Can you work these out from the model? Positions are in its coordinate system, mm. Coordinates: 2 decimals unless noted, no trailing zeros. Loops run counter-clockwise (first coordinate to the right, second up) from the corner with the lowest first, then second, coordinate; pieces in that order, holes last.
```python
from build123d import *

# Parameters (mm, degrees)
FILLET2_R = 10


# Read off the part's stored shape, not the designer's step: Revolve-Thin1
with BuildPart() as part:
    # Revolve-Thin1 outline → Revolve-Thin1 (revolve)
    with BuildSketch(Plane.YX):
        with BuildLine():
            ThreePointArc((20.809194043, 175.40901311), (18.540551824, 164.003778488), (17.78, 152.4))
            ThreePointArc((17.78, 152.4), (18.931985096, 144.91543265), (22.281305618, 138.123682499))
            ThreePointArc((22.281305618, 138.123682499), (40.863057404, 136.154543576), (50.8, 120.33))
            Line((50.8, 120.33), (50.8, 0))
            Line((50.8, 0), (53.34, 0))
            Line((53.34, 0), (53.34, 120.464002572))
            ThreePointArc((53.34, 120.464002572), (43.123071275, 137.708761877), (23.372253336, 141.125272789))
            ThreePointArc((23.372253336, 141.125272789), (21.096554077, 146.559714816), (20.32, 152.4))
            ThreePointArc((20.32, 152.4), (21.058821772, 163.67224196), (23.262645642, 174.751612735))
            add(Edge.make_bspline(
                [(23.262645642, 174.751612735), (35.023141074, 218.642379212), (41.79057094, 257.222392684), (43.53651902, 290.537066698)],
                knots=[0, 0, 0, 0, 1, 1, 1, 1], degree=3))
            Line((43.53651902, 290.537066698), (41.000000001, 290.670000027))
            add(Edge.make_bspline(
                [(41.000000001, 290.670000027), (38.399983722, 241.058733938), (20.809194043, 175.40901311)],
                knots=[0.495939659, 0.495939659, 0.495939659, 0.498282386, 0.498282386, 0.498282386], degree=2))
        make_face()
    revolve(axis=Axis((0, 0, 0), (1, 0, 0)))

    # Fillet2
    fillet2_edges = [part.edges().sort_by_distance(p)[0] for p in [
        (138.123682499, -22.281305618, 0),
        (120.33, -50.8, 0),
        (120.464002572, -53.34, 0),
        (141.125272789, -23.372253336, 0),
    ]]
    fillet(fillet2_edges, radius=FILLET2_R)


solid = part.part
```
(1) If I drill on probe 1 along Z at (x, y) = (31.5, 0); probe 2 along Z at (x, y) = (267.5, 34.5), over which ranges is the centre line in solid material (lowest first)?
Check values:
probe 1: z = -53.34 to -50.8, 50.8 to 53.34
probe 2: z = -23.29 to -18.33, 18.33 to 23.29
(2) I want a section at A-A on x = 58.5. Write out the boundary of the cut face in (y, z), then the cut area to 3 significant figures.
Check values:
outline: circle Ø106.68 at (0, 0); hole circle Ø101.6 at (0, 0)
area: 831 mm2
(3) I'm going to push flat-ended pins straight in: pin 1 (1 mm diameter, centred on x = 67, y = 1.5, fed in from -Z); pin 2 (2 mm diameter, centred on y = 16.5, z = 28, fed in from -X); pin 3 (1 mm diameter, centred on y = -19, z = -8, fed in from -X). Where does each tip first touch, or does it pass through?
Check values:
pin 1: stops at z = -53.33
pin 2: stops at x = 139.03
pin 3: stops at x = 142.2
(4) I want a section at B-B on x = 131.5. Write out the boundary of the cut face in (y, z), then the cut area to 3 significant figures.
Check values:
outline: circle Ø98.61 at (0, 0); hole circle Ø92.27 at (0, 0)
area: 949 mm2
(5) If we mould it in two halves opening along Y, with no side actions, what happens to faces 1 (the cylindrical face through (59.013, 48.454, 15.259)), 2 (the cylindrical face through (60.78, -6.944, 52.886)), 3 (the flat face through (0, -47, -20))? For each: released by +Y, released by -Y, zero draft, split by the parting line, or undercut.
Check values:
face 1: undercut
face 2: split by the parting line
face 3: zero draft
